The listing builds one solid part. Answer for the finished solid, in the listing's coordinates (mm). Face numbers are marked on the shaded views. A direction names the side the tool comes from. Coordinates: 2 decimals unless noted, no trailing zeros. Return JSON: item names as keys, results as strings.
```python
from build123d import *
from OCP.BRepFilletAPI import BRepFilletAPI_MakeChamfer

# Parameters (mm, degrees)
SKETCH1_W               = 45
SKETCH1_H               = 70
BOSS_EXTRUDE1_DEPTH     = 18
CUT_EXTRUDE1_DEPTH      = 60.782940711
CUT_EXTRUDE1_DEPTH_BACK = 60.782940711
SKETCH2_W               = 20.25
SKETCH2_H               = 9.5
SKETCH3_R               = 4.2
CUT_EXTRUDE2_DEPTH      = 46.33486517
FILLET1_R               = 10
CUT_EXTRUDE3_DEPTH      = 46.33486517
FILLET2_R               = 8
FILLET4_R               = 2
CHAMFER1_SIZE           = 0.5
CHAMFER1_SIZE2          = 1.37373871


with BuildPart() as part:
    # Sketch1 → Boss-Extrude1 (new body)
    with BuildSketch(Plane(origin=(0, 0, 0), x_dir=(1, 0, 0), z_dir=(0, 1, 0))):
        Rectangle(SKETCH1_W, SKETCH1_H)
    extrude(amount=BOSS_EXTRUDE1_DEPTH)

    # Sketch2 → Cut-Extrude1 (cut, two sides: drawn at the far end of the back side and taken through both)
    with BuildSketch(Plane(origin=(22.5, 0, 0), x_dir=(0, 0, -1), z_dir=(1, 0, 0)).offset(-CUT_EXTRUDE1_DEPTH_BACK)):
        with Locations((0, 4.75)):
            Rectangle(SKETCH2_W, SKETCH2_H)
    extrude(amount=CUT_EXTRUDE1_DEPTH + CUT_EXTRUDE1_DEPTH_BACK, mode=Mode.SUBTRACT)

    # Sketch3 → Cut-Extrude2 (cut, through all)
    with BuildSketch(Plane.XZ):
        with Locations(Location((15, 25, 0), (0, 0, 270))):
            Circle(SKETCH3_R)
        with Locations(Location((15, -25, 0), (0, 0, 270))):
            Circle(SKETCH3_R)
        with Locations(Location((-15, -25, 0), (0, 0, 270))):
            Circle(SKETCH3_R)
        with Locations(Location((-15, 25, 0), (0, 0, 270))):
            Circle(SKETCH3_R)
    extrude(amount=-CUT_EXTRUDE2_DEPTH, mode=Mode.SUBTRACT)

    # Fillet1
    fillet1_edges = [part.edges().sort_by_distance(p)[0] for p in [
        (-22.5, 9, -35),
        (22.5, 9, -35),
        (22.5, 9, 35),
        (-22.5, 9, 35),
    ]]
    fillet(fillet1_edges, radius=FILLET1_R)

    # Sketch6 → Cut-Extrude3 (cut, through all)
    with BuildSketch(Plane.XZ):
        with BuildLine():
            Line((12.5, 35), (-12.5, 35))
            ThreePointArc((-12.5, 35), (0, 33.26906369), (12.5, 35))
        make_face()
        with BuildLine():
            Line((12.5, -35), (-12.5, -35))
            ThreePointArc((-12.5, -35), (0, -33.26906369), (12.5, -35))
        make_face()
    extrude(amount=-CUT_EXTRUDE3_DEPTH, mode=Mode.SUBTRACT)

    # Fillet2
    fillet2_edges = [part.edges().sort_by_distance(p)[0] for p in [
        (12.5, 9, 35),
        (-12.5, 9, 35),
        (12.5, 9, -35),
        (-12.5, 9, -35),
    ]]
    fillet(fillet2_edges, radius=FILLET2_R)

    # Fillet4
    fillet4_edges = [part.edges().sort_by_distance(p)[0] for p in [
        (-22.5, 18, 0),
        (22.5, 18, 0),
        (20.63102045, 18, -30.821211768),
        (-20.63102045, 18, 30.821211768),
        (0, 18, 33.26906369),
        (20.63102045, 18, 30.821211768),
        (0, 18, -33.26906369),
        (-20.63102045, 18, -30.821211768),
        (13.473401565, 18, -34.886533438),
        (-13.473401565, 18, -34.886533438),
        (-13.473401565, 18, 34.886533438),
        (13.473401565, 18, 34.886533438),
    ]]
    fillet(fillet4_edges, radius=FILLET4_R)

    # Chamfer1: one chamfer whose edges measure the first distance from different faces: ONE call of the kernel's chamfer builder (chamfer() names one face for all edges)
    chamfer1_edges_1 = [part.edges().sort_by_distance(p)[0] for p in [
        (-15, 0, -20.8),
        (15, 0, -20.8),
    ]]
    chamfer1_side_1 = [part.faces().sort_by_distance(p)[0] for p in [
        (0, 0, -21.437561791),
    ]]
    chamfer1_edges_2 = [part.edges().sort_by_distance(p)[0] for p in [
        (-15, 0, 29.2),
        (15, 0, 29.2),
    ]]
    chamfer1_side_2 = [part.faces().sort_by_distance(p)[0] for p in [
        (0, 0, 21.437561791),
    ]]
    chamfer1 = BRepFilletAPI_MakeChamfer(part.part.solid().wrapped)
    for e in chamfer1_edges_1:
        chamfer1.Add(CHAMFER1_SIZE, CHAMFER1_SIZE2, e.wrapped, chamfer1_side_1[0].wrapped)  # the first distance lies on this face
    for e in chamfer1_edges_2:
        chamfer1.Add(CHAMFER1_SIZE, CHAMFER1_SIZE2, e.wrapped, chamfer1_side_2[0].wrapped)  # the first distance lies on this face
    add(Compound.cast(chamfer1.Shape()), mode=Mode.REPLACE)


solid = part.part
```
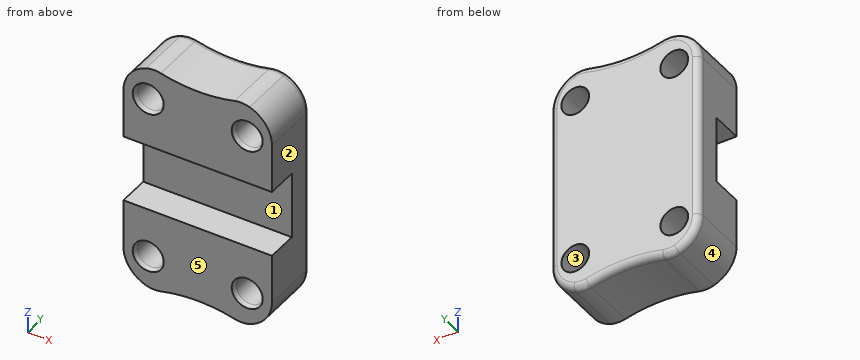
Item 1: Which of the six approach directions +Z, -Z, +X, -X, +Y, -Y give full straight-line access (tool end or side, diameter ignored) to the marked faces 1 and 2?
Answer list:
{"face 1": "+X, -X, -Y", "face 2": "+Z, -Z, +X, +Y, -Y"}
Item 2: Find the intervals of material crossed by probe 1 along X at (y, z) = (10.5, 25); probe 2 along Z at (x, y) = (15.5, 5.5) (3 decimals); probe 3 along X at (y, z) = (6, 24), in increasing order.
Answer list:
{"probe 1": "-22.5 to -19.2, -10.8 to 10.8, 19.2 to 22.5", "probe 2": "-34.539 to -29.17, -20.83 to -10.125, 10.125 to 20.83, 29.17 to 34.539", "probe 3": "-22.5 to -19.08, -10.92 to 10.92, 19.08 to 22.5"}
Item 3: Determine the mould class of the marked faces 3, 4 and 5 for opening direction X: pulls with the +X half, pulls with the -X half, needs draft (parallel to the pull), parting line crosses it, or undercut.
Answer list:
{"face 3": "undercut", "face 4": "pulls with the -X half", "face 5": "needs draft"}
Item 4: Flat-ended cylindrical pins translate along their axes: pin 1 (10 mm diameter, centred on x = -3.5, z = -0.5, fed in from -Y); pin 2 (4 mm diameter, centred on x = 8, y = 15.5, fed in from -Z); pin 3 (5 mm diameter, centred on x = -8.5, y = 3, fed in from -Z). Find the tip coordinate at first contact, or state that the pin passes through.
Answer list:
{"pin 1": "y = 9.5", "pin 2": "z = -34.37", "pin 3": "z = -34.6"}
Item 5: The part is cut by section A-A on y = 12.75. Count the separate pieces of the cut face and the enclosed holes in it, plus the area to 3 significant figures.
Answer list:
{"separate pieces": "1", "enclosed holes": "4", "area": "2,780 mm2"}
